Part model, mm, in its own coordinate system. Face numbers are marked on the shaded views. A direction names the side the tool comes from. Coordinates: 2 decimals unless noted, no trailing zeros. Write each loop counter-clockwise with the first axis right and the second up, starting at its lowest first coordinate (ties: lowest second). Pieces come first, ordered by that corner, then holes. Notation, with made-up numbers: (16.5, -19.5) -> (54.5, -19.5) arc R13 cw to (54.5, 5.5) -> close; hole circle Ø6 at (-15, 53.25). An arc over 180 degrees is marked (long way). One line per question, with ' | ' between items. Start each with the question number.
Item 1: 3-axis set-ups, long thin cutter, end or side, ignore diameter. For the marked faces 4 and 5: which of +Z, -Z, +X, -X, +Y, -Y reach the whole face in a straight line?
Item 2: Saw through at C-C (y = -1.5). List the corners of the cut face in (x, z).
Item 3: Probe probe 1 along Z at (x, y) = (0, 1.2); probe 2 along X at (y, z) = (0.9, 0); probe 3 along X at (y, z) = (6, 4.5). List the from-to ranges inside material, lowest first. Write a range as [from, to].
Item 4: Saw through at A-A (y = -6). List the corners of the cut face in (x, z), and give its area (3 significant figures).
Item 5: Two-plate mould, pull along Y, no slides. Class the marked faces 1, 2 and 3: pulls with the +Y half, pulls with the -Y half, needs draft (parallel to the pull), parting line crosses it, or undercut.
Item 6: Saw through at B-B (z = 0). List the corners of the cut face in (x, y), and give its area (3 significant figures).
Item 7: Pin check, flat tips, straight feed: pin 1 (6 mm diameter, centred on x = 0.5, y = -24, fed in from +Z); pin 2 (1.5 mm diameter, centred on x = 2, y = -3, fed in from -Z); pin 3 (2 mm diameter, centred on x = 5.5, y = -7, fed in from -Z). Stop position of each tip, or through.
from build123d import *

# Parameters (mm, degrees)
BOSS_EXTRUDE1_DEPTH = 8
SKETCH2_R           = 5
BOSS_EXTRUDE2_DEPTH = 28
FILLET1_R           = 2
SKETCH3_R           = 1.55
CUT_EXTRUDE1_DEPTH  = 15.6
FILLET2_R           = 1
SKETCH5_R           = 1.6
CUT_EXTRUDE3_DEPTH  = 4
SKETCH6_R           = 0.5
CUT_EXTRUDE4_DEPTH  = 0.5
CUT_EXTRUDE5_REACH  = 10
SKETCH7_R           = 1


with BuildPart() as part:
    # Sketch1 → Boss-Extrude1 (new body)
    with BuildSketch(Plane(origin=(0, 0, 0), x_dir=(1, 0, 0), z_dir=(0, 1, 0))):
        Polygon((7.3, -4.214656965), (7.3, 4.214656965), (0, 8.42931393), (-7.3, 4.214656965), (-7.3, -4.214656965), (0, -8.42931393), align=None)
    extrude(amount=BOSS_EXTRUDE1_DEPTH)

    # Sketch2 → Boss-Extrude2 (add)
    with BuildSketch(Plane.XZ):
        Circle(SKETCH2_R)
        with BuildLine():
            Line((-1.15, 1.112429773), (-1.15, -1.112429773))
            ThreePointArc((-1.15, -1.112429773), (1.6, 0), (-1.15, 1.112429773))
        make_face(mode=Mode.SUBTRACT)
    extrude(amount=BOSS_EXTRUDE2_DEPTH)

    # Fillet1
    fillet1_edges = [part.edges().sort_by_distance(p)[0] for p in [
        (-5, 0, 0),
    ]]
    fillet(fillet1_edges, radius=FILLET1_R)

    # Sketch3 → Cut-Extrude1 (cut, through all)
    with BuildSketch(Plane(origin=(7.3, 0, 0), x_dir=(0, 0, -1), z_dir=(1, 0, 0))):
        with Locations((-0.085343035, 3.85)):
            Circle(SKETCH3_R)
    extrude(amount=-CUT_EXTRUDE1_DEPTH, mode=Mode.SUBTRACT)

    # Fillet2
    fillet2_edges = [part.edges().sort_by_distance(p)[0] for p in [
        (0, 4, 8.42931393),
        (-7.3, 4, 4.214656965),
        (-7.3, 4, -4.214656965),
        (0, 4, -8.42931393),
        (7.3, 4, -4.214656965),
        (7.3, 4, 4.214656965),
        (3.65, 8, -6.321985448),
        (-3.65, 8, -6.321985448),
        (-7.3, 8, 0),
        (-3.65, 8, 6.321985448),
        (3.65, 8, 6.321985448),
        (7.3, 8, 0),
    ]]
    fillet(fillet2_edges, radius=FILLET2_R)

    # Sketch5 → Cut-Extrude3 (cut)
    with BuildSketch(Plane.XZ.offset(28)):
        Circle(SKETCH5_R)
    extrude(amount=-CUT_EXTRUDE3_DEPTH, mode=Mode.SUBTRACT)

    # Sketch6 → Cut-Extrude4 (cut)
    with BuildSketch(Plane(origin=(-3.65, 0, 6.321985448), x_dir=(0.866025404, 0, 0.5), z_dir=(-0.5, 0, 0.866025404))):
        with Locations((-1.5, 3.5)):
            Circle(SKETCH6_R)
        with Locations((1.5, 3.5)):
            Circle(SKETCH6_R)
    extrude(amount=-CUT_EXTRUDE4_DEPTH, mode=Mode.SUBTRACT)

    # Sketch7 → Cut-Extrude5 (cut, up to next)
    with BuildSketch(Plane.XZ, mode=Mode.PRIVATE) as cut_extrude5_sk1:
        Circle(SKETCH7_R)
    cut_extrude5_tool1 = extrude(cut_extrude5_sk1.sketch, amount=-CUT_EXTRUDE5_REACH, mode=Mode.PRIVATE) & part.part
    add(cut_extrude5_tool1.solids().sort_by_distance((0, 0, 0))[0], mode=Mode.SUBTRACT)


solid = part.part
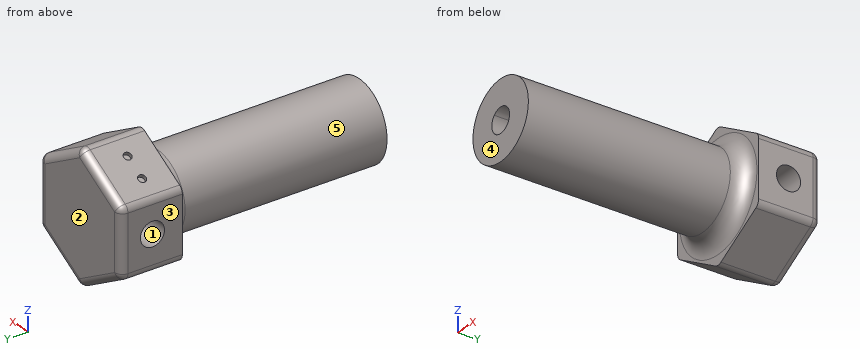
From the geometry:
1) face 4: +Z, -Z, +X, -X, -Y | face 5: -Y
2) outline: circle Ø10.13 at (0, 0); hole (-1.15, -1.11) arc R1.6 ccw (long way) to (-1.15, 1.11) -> close
3) probe 1: [-8.27, -1], [1, 8.27] | probe 2: [-7.3, -1], [1, 7.3] | probe 3: [-6.81, 6.81]
4) outline: circle Ø10 at (0, 0); hole (-1.15, -1.11) arc R1.6 ccw (long way) to (-1.15, 1.11) -> close | area: 71.2 mm2
5) face 1: undercut | face 2: pulls with the +Y half | face 3: needs draft
6) outline: (-7.3, 0) -> (-7, 0) arc R2 cw to (-5, -2) -> (-5, -28) -> (-1.6, -28) -> (-1.6, -24) -> (-1.15, -24) -> (-1.15, 0) -> (-1, 0) -> (-1, 2.3) -> (-7.3, 2.3) -> close; (-7.3, 5.4) -> (7.3, 5.4) -> (7.3, 7) arc R1 ccw to (6.3, 8) -> (-6.3, 8) arc R1 ccw to (-7.3, 7) -> close; (1, 0) -> (1.6, 0) -> (1.6, -28) -> (5, -28) -> (5, -2) arc R2 cw to (7, 0) -> (7.3, 0) -> (7.3, 2.3) -> (1, 2.3) -> close | area: 269 mm2
7) pin 1: z = 5 | pin 2: z = -4.84 | pin 3: z = -2.18
